Geometry: see drawing. Coordinates: mm, zero at the bounding-box minimum. Round coordinates to 2 decimals unless told otherwise and drop trailing zeros. Order: outer loops, then holes, each group sorted by start corner. A loop starts at its lowest first (then second) coordinate and runs counter-clockwise, first axis right, second up. Notation, with made-up numbers: (89, 70.5) - (120, 70.5) arc R19 cw to (120, 79.5) - close; hole circle Ø1 at (64.25, 21). An arc over 180 degrees is marked (long way). Put each result on its own line as item: value. Start each with the question number.
1) Section B-B on x = 5. Output: boundary loops of the cut face in (y, z), then the cut area to 3 significant figures.
2) Section D-D on x = 0.75. Output: boundary loops of the cut face in (y, z), then the cut area to 3 significant figures.
3) Section A-A on z = 40. Output: boundary loops of the cut face in (x, y).
4) Contact query for flat-ended pins moving along their axis: P1, Ø6, axis at x = 8, z = 43.5, coming from the -Y side; P2, Ø4, axis at x = 6.5, z = 58.5, coming from the +Y side. Output: stop coordinate, or through.
5) Section C-C on y = 3.5. Output: boundary loops of the cut face in (x, z), then the cut area to 3 significant figures.
6) Line query: probe 1 along Z at (x, y) = (5, 3.75); probe 2 along X at (y, z) = (10.5, 77); probe 3 along Z at (x, y) = (5, 7.25). Output: solid intervals per line, ascending. Write a range as [from, to].
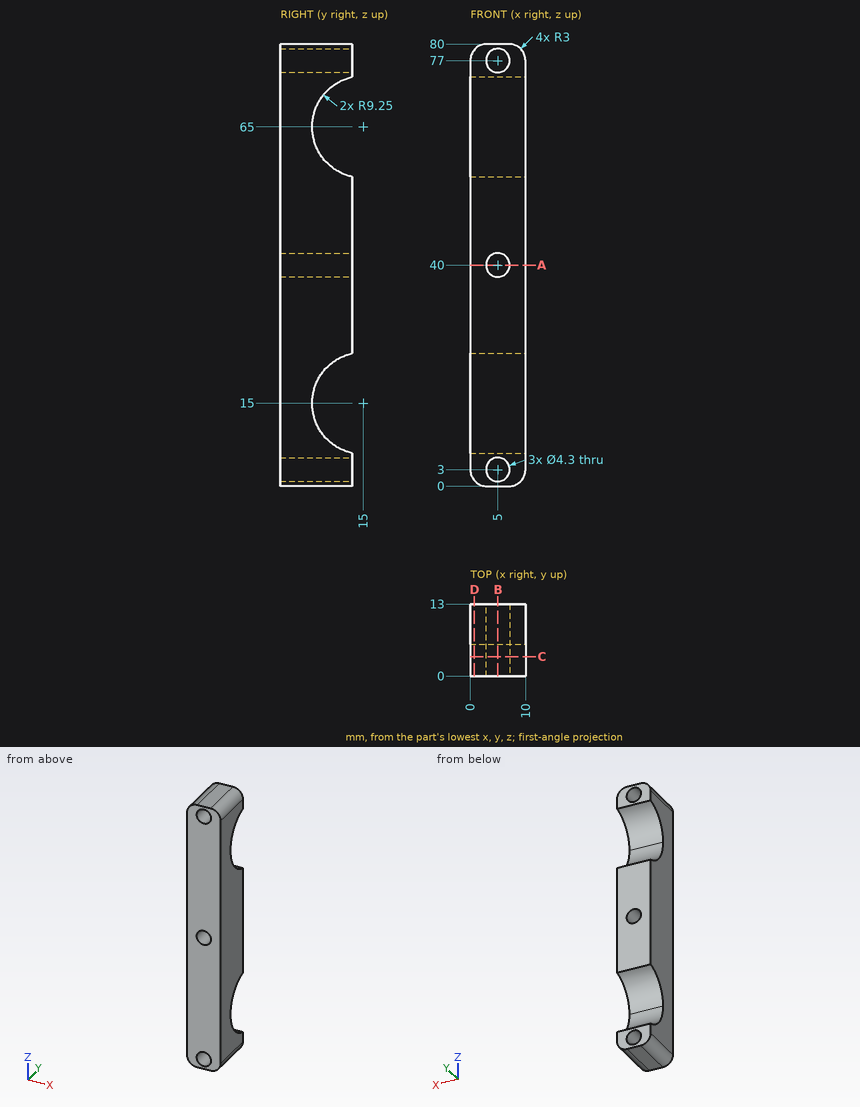
Answer sheet:
1. outline: (0, 0) - (13, 0) - (13, 0.85) - (0, 0.85) - close; (0, 5.15) - (13, 5.15) - (13, 5.97) arc R9.25 cw to (13, 24.03) - (13, 37.85) - (0, 37.85) - close; (0, 42.15) - (13, 42.15) - (13, 55.97) arc R9.25 cw to (13, 74.03) - (13, 74.85) - (0, 74.85) - close; (0, 79.15) - (13, 79.15) - (13, 80) - (0, 80) - close
1. area: 677 mm^2
2. outline: (0, 1.02) - (13, 1.02) - (13, 5.97) arc R9.25 cw to (13, 24.03) - (13, 55.97) arc R9.25 cw to (13, 74.03) - (13, 78.98) - (0, 78.98) - close
2. area: 818 mm^2
3. outline: (0, 0) - (2.85, 0) - (2.85, 13) - (0, 13) - close; (7.15, 0) - (10, 0) - (10, 13) - (7.15, 13) - close
4. P1: y = 0
4. P2: y = 11.35
5. outline: (0, 3) arc R3 ccw to (3, 0) - (7, 0) arc R3 ccw to (10, 3) - (10, 77) arc R3 ccw to (7, 80) - (3, 80) arc R3 ccw to (0, 77) - close; hole circle Ø4.3 at (5, 3); hole circle Ø4.3 at (5, 40); hole circle Ø4.3 at (5, 77)
5. area: 749 mm^2
6. probe 1: [0, 0.85], [5.15, 37.85], [42.15, 74.85], [79.15, 80]
6. probe 2: [0, 2.85], [7.15, 10]
6. probe 3: [0, 0.85], [5.15, 9.95], [20.05, 37.85], [42.15, 59.95], [70.05, 74.85], [79.15, 80]
